```python
from build123d import *

# Parameters (mm, degrees)
BOSS_EXTRUDE1_DEPTH = 42
BOSS_EXTRUDE3_DEPTH = 16
SKETCH7_R           = 10
CUT_EXTRUDE2_DEPTH  = 16
BOSS_EXTRUDE4_DEPTH = 16
SKETCH9_R           = 12
CUT_EXTRUDE3_DEPTH  = 16
FILLET1_R           = 21
BOSS_EXTRUDE5_DEPTH = 16
SKETCH12_R          = 10
CUT_EXTRUDE5_DEPTH  = 16


with BuildPart() as part:
    # Sketch2 → Boss-Extrude1 (new, symmetric)
    with BuildSketch(Plane(origin=(0, 0, 0), x_dir=(0, 0, -1), z_dir=(1, 0, 0))):
        Polygon((0, 0), (-134, 0), (-134, -16), (16, -16), (16, 12), (84, 12), (84, 28), (0, 28), align=None)
    extrude(amount=BOSS_EXTRUDE1_DEPTH, both=True)

    # Sketch6 → Boss-Extrude3 (add)
    with BuildSketch(Plane.XY):
        with BuildLine():
            Line((-67.990788091, 71.168031394), (-42, 28))
            Line((-42, 28), (42, 28))
            Line((42, 28), (-36.012593074, 97.663730318))
            ThreePointArc((-36.012593074, 97.663730318), (-63.398219306, 98.170581914), (-67.990788091, 71.168031394))
        make_face()
    extrude(amount=-BOSS_EXTRUDE3_DEPTH)

    # Sketch7 → Cut-Extrude2 (cut)
    with BuildSketch(Plane.XY):
        with Locations((-50, 82)):
            Circle(SKETCH7_R)
    extrude(amount=-CUT_EXTRUDE2_DEPTH, mode=Mode.SUBTRACT)

    # Sketch8 → Boss-Extrude4 (add)
    with BuildSketch(Plane(origin=(0, 28, 0), x_dir=(1, 0, 0), z_dir=(0, 1, 0))):
        with BuildLine():
            Line((-12, 114), (58, 114))
            ThreePointArc((58, 114), (88, 84), (58, 54))
            Line((58, 54), (-12, 54))
            ThreePointArc((-12, 54), (-42, 84), (-12, 114))
        make_face()
    extrude(amount=-BOSS_EXTRUDE4_DEPTH)

    # Sketch9 → Cut-Extrude3 (cut)
    with BuildSketch(Plane(origin=(0, 28, 0), x_dir=(1, 0, 0), z_dir=(0, 1, 0))):
        with Locations(Location((-12, 84, 0), (0, 0, 270))):
            Circle(SKETCH9_R)
        with Locations(Location((58, 84, 0), (0, 0, 270))):
            Circle(SKETCH9_R)
    extrude(amount=-CUT_EXTRUDE3_DEPTH, mode=Mode.SUBTRACT)

    # Fillet1
    fillet1_edges = [part.edges().sort_by_distance(p)[0] for p in [
        (42, 20, -54),
    ]]
    fillet(fillet1_edges, radius=FILLET1_R)

    # Sketch11 → Boss-Extrude5 (add)
    with BuildSketch(Plane.XY.offset(134)):
        with BuildLine():
            Line((0, 61), (0, 0))
            Line((0, 0), (42, 0))
            Line((42, 0), (42, 82))
            ThreePointArc((42, 82), (35.849242405, 96.849242405), (21, 103))
            Line((21, 103), (-49, 103))
            ThreePointArc((-49, 103), (-70, 82), (-49, 61))
            Line((-49, 61), (0, 61))
        make_face()
    extrude(amount=-BOSS_EXTRUDE5_DEPTH)

    # Sketch12 → Cut-Extrude5 (cut)
    with BuildSketch(Plane.XY.offset(134)):
        with Locations((-49, 82)):
            Circle(SKETCH12_R)
        with Locations((21, 82)):
            Circle(SKETCH12_R)
    extrude(amount=-CUT_EXTRUDE5_DEPTH, mode=Mode.SUBTRACT)


solid = part.part
```
Read the model definition and answer for the solid it produces. Units are mm, in the model's axes. A direction names the side the tool comes from. Coordinates: 2 decimals unless noted, no trailing zeros. Write each loop counter-clockwise with the first axis right and the second up, starting at its lowest first coordinate (ties: lowest second). Pieces come first, ordered by that corner, then holes. Notation, with made-up numbers: (-29, 71) -> (15, 71) arc R17 ccw to (15, 103) -> close; hole circle Ø4 at (66.5, -26). An arc over 180 degrees is marked (long way). Write item = value, one per line.
(1) Section A-A on x = -19 is taken. Write down the section's boundary in (y, z), plus the area to 3 significant figures.
From the geometry:
outline = (-16, -16) -> (12, -16) -> (12, -74.25) -> (28, -74.25) -> (28, -16) -> (82.47, -16) -> (82.47, 0) -> (0, 0) -> (0, 134) -> (-16, 134) -> close; (12, -113.17) -> (28, -113.17) -> (28, -93.75) -> (12, -93.75) -> close; (61, 118) -> (103, 118) -> (103, 134) -> (61, 134) -> close
area = 5,630 mm2
(2) Straight lines are drawn through the part: L1, parallel to Z at x = 12, y = 53; L2, parallel to Y at x = -49, z = 130.25; L3, parallel to Y at x = 21, z = 128. For each, find the intervals that lie inside material, in ascending order. Write a range as from..to.
From the geometry:
L1 = -16..0, 118..134
L2 = 61..72, 92..103
L3 = -16..72, 92..103
(3) Section B-B on y = 46 is taken. Write down the section's boundary in (x, z).
From the geometry:
outline = (-52.84, -16) -> (21.84, -16) -> (21.84, 0) -> (-52.84, 0) -> close; (0, 118) -> (42, 118) -> (42, 134) -> (0, 134) -> close
(4) Given pin 1 Ø8 at (y, z) = (37, 125.5) entering from -X; pin 2 Ø12 at (x, y) = (8.5, -2.5) entering from -Z; pin 3 Ø12 at (x, z) = (15.5, -83.5) entering from +Y, each flat-ended and moving along its own axis, determine where each tip first touches the part or whether it passes through.
From the geometry:
pin_1 = 0
pin_2 = -16
pin_3 = 28
(5) Which of the six approach directions +Z, -Z, +X, -X, +Y, -Y give full straight-line access (tool end or side, diameter ignored) to faces 5 (the face through (-70, 82, 126)), 6 (the face through (9, 12, -66)), 7 (the face through (-50.302, 91.915, 126.112)), 8 (the face through (-28, 58, -16)), 9 (the face through (-2, 64, 118))?
From the geometry:
face_5 = +Z, -X
face_6 = -Z, +X, -X, -Y
face_7 = +Z
face_8 = -Z, +X, -X, +Y
face_9 = +X, -X, +Y
(6) For a pull along Y with two mould halves and no side action, classify faces 1 (the face through (-51.302, 91.915, -7.888)), 2 (the face through (0, 31, 126)), 3 (the face through (-63.074, 98.434, -7.888)), 4 (the face through (23, 20, -114)) as +Y half, -Y half, draft (parallel to the pull), parting line (faces both ways), or undercut.
From the geometry:
face_1 = undercut
face_2 = undercut
face_3 = parting line
face_4 = draft
(7) Section D-D on z = -28 is taken. Write down the section's boundary in (x, y), plus the area to 3 significant figures.
From the geometry:
outline = (-42, 12) -> (42, 12) -> (42, 28) -> (-42, 28) -> close
area = 1,340 mm2
(8) Section C-C on y = 31.5 is taken. Write down the section's boundary in (x, z).
From the geometry:
outline = (-44.11, -16) -> (38.08, -16) -> (38.08, 0) -> (-44.11, 0) -> close; (0, 118) -> (42, 118) -> (42, 134) -> (0, 134) -> close
